```python
from build123d import *

# Parameters (mm, degrees)
SKETCH1_R          = 1.7526
EXTRUDE1_DEPTH     = 12.7
CHAMFER3_SIZE      = 0.5953125
SKETCH6_R          = 2.8702
EXTRUDE2_DEPTH     = 3.5052
CUT_EXTRUDE1_DEPTH = 2.08359375
CHAMFER1_SIZE      = 0.28702
CHAMFER2_SIZE      = 0.14351


with BuildPart() as part:
    # Sketch1 → Extrude1 (new body)
    with BuildSketch(Plane.XY):
        Circle(SKETCH1_R)
    extrude(amount=-EXTRUDE1_DEPTH)

    # Chamfer3
    chamfer3_edges = [part.edges().sort_by_distance(p)[0] for p in [
        (-1.7526, 0, 0),
    ]]
    chamfer(chamfer3_edges, length=CHAMFER3_SIZE)

    # Sketch6 → Extrude2 (add)
    with BuildSketch(Plane(origin=(0, 0, -12.7), x_dir=(-1, 0, 0), z_dir=(0, 0, -1))):
        Circle(SKETCH6_R)
    extrude(amount=EXTRUDE2_DEPTH)

    # Sketch7 → Cut-Extrude1 (cut)
    with BuildSketch(Plane(origin=(0, 0, -16.2052), x_dir=(-1, 0, 0), z_dir=(0, 0, -1))):
        Polygon((0, 1.603951217), (-1.3890625, 0.801975608), (-1.3890625, -0.801975608), (0, -1.603951217), (1.3890625, -0.801975608), (1.3890625, 0.801975608), align=None)
    extrude(amount=-CUT_EXTRUDE1_DEPTH, mode=Mode.SUBTRACT)

    # Cut-Extrude2 cone 1 section (through the dimple's axis) → Cut-Extrude2 (revolve, cut)
    with BuildSketch(Plane(origin=(0, 0, -16.2052), x_dir=(0, 1, 0), z_dir=(1, 0, 0))):
        Polygon((0, 0), (1.603951217, 0), (0, 1.603951217), align=None)
    revolve(axis=Axis((0, 0, -16.2052), (0, 0, 1)), mode=Mode.SUBTRACT)

    # Chamfer1
    chamfer1_edges = [part.edges().sort_by_distance(p)[0] for p in [
        (2.8702, 0, -16.2052),
    ]]
    chamfer(chamfer1_edges, length=CHAMFER1_SIZE)

    # Chamfer2
    chamfer2_edges = [part.edges().sort_by_distance(p)[0] for p in [
        (2.8702, 0, -12.7),
    ]]
    chamfer(chamfer2_edges, length=CHAMFER2_SIZE)


solid = part.part
```
Source: CAD feature listing. Evaluate the final solid. Frame: model axes, mm. A direction names the side the tool comes from. Coordinates: 2 decimals unless noted, no trailing zeros. Order: outer loops, then holes, each group sorted by start corner. A loop starts at its lowest first (then second) coordinate and runs counter-clockwise, first axis right, second up. Notation, with made-up numbers: (79.5, -24.75) - (109.5, -24.75) arc R18 cw to (109.5, 3.25) - close; hole circle Ø5 at (-34, -5.75). An arc over 180 degrees is marked (long way). One line per item, written item: value.
1) Cut plane A-A on y = 0. Output: boundary loops of the cut face in (x, z).
Computed values:
outline: (-2.87, -15.92) - (-2.58, -16.21) - (-1.6, -16.21) - (-1.39, -15.99) - (-1.39, -14.12) - (1.39, -14.12) - (1.39, -15.99) - (1.6, -16.21) - (2.58, -16.21) - (2.87, -15.92) - (2.87, -12.84) - (2.73, -12.7) - (1.75, -12.7) - (1.75, -0.6) - (1.16, 0) - (-1.16, 0) - (-1.75, -0.6) - (-1.75, -12.7) - (-2.73, -12.7) - (-2.87, -12.84) - close
2) Contact query for flat-ended pins moving along their axis: pin 1 (2 mm diameter, centred on y = -1.5, z = -13, fed in from -X); pin 2 (0.5 mm diameter, centred on y = 0.5, z = -15.5, fed in from -X); pin 3 (2 mm diameter, centred on x = -1.5, y = 2, fed in from +Z). Output: stop coordinate, or through.
Computed values:
pin 1: stops at x = -2.83
pin 2: stops at x = -2.86
pin 3: stops at z = -0.34
3) Mould query, pull axis X, two halves, no side actions, for faces 4 (the face through (2.278, -1.746, -14.359)), 5 (the face through (-1.389, 0, -15)), 6 (the face through (0, 0, -14.122)), 7 (the face through (0, -2, -12.7)). Classes: released by +X, released by -X, zero draft, split by the parting line, or undercut.
Computed values:
face 4: split by the parting line
face 5: undercut
face 6: undercut
face 7: zero draft
4) Cut plane B-B on z = -10.5. Output: boundary loops of the cut face in (x, y).
Computed values:
outline: circle Ø3.51 at (0, 0)
5) Cut plane C-C on z = -13. Output: boundary loops of the cut face in (x, y), plus the area to 3 significant figures.
Computed values:
outline: circle Ø5.74 at (0, 0)
area: 25.9 mm^2
6) Ray query, line 1 (Z direction, x = -2.05, y = 0.65); line 2 (Z direction, x = -0.55, y = 0.95); line 3 (Y direction, x = -1.15, z = -7.75). Return the intervals inside material, ascending. Write a range as [from, to].
Computed values:
line 1: z = [-16.21, -12.7]
line 2: z = [-14.12, 0]
line 3: y = [-1.32, 1.32]
7) Reachability of faces 1 (the face through (0.7, -1.2, -15.2)), 2 (the face through (1.67, 0.53, -6.56)), 3 (the face through (-2, 0, -16.205)) from +Z, -Z, +X, -X, +Y, -Y: full face, straight path, thin tool, end or side. Return the list, or none.
Computed values:
face 1: -Z
face 2: +Z
face 3: -Z, +X, -X, +Y, -Y
